The model under review builds one solid part; all positions refer to its coordinate system, in mm. A direction names the side the tool comes from. Round coordinates to 2 decimals unless told otherwise and drop trailing zeros. Order: outer loops, then holes, each group sorted by start corner. A loop starts at its lowest first (then second) coordinate and runs counter-clockwise, first axis right, second up. Notation, with made-up numbers: M 37.5,32.25 L 71.5,32.25 A24 ccw 71.5,53.25 Z; hole C 85,73 d9. An arc over 180 degrees is marked long. Answer as a JSON object with one key per item and string values. Group by question number.
1. Add section A-A on z = 5. State the section outline as (x, y) points, and give its area (3 significant figures).
2. Mouldability with a two-part tool opening along Z and no side actions: class faces 1 (the face through (-16.297, 39.418, 4.934)), 2 (the face through (-28.295, 36.978, 5.07)), 3 (the face through (-30.8, -25.9, 1.5)), 4 (the face through (-31.2, -24.2, 3.5)) as released by +Z, released by -Z, zero draft, split by the parting line, or undercut.
3. Machinability: for faces 5 (the face through (-30.8, -25.9, 8.5)), 6 (the face through (-29.799, 1, 5)), 7 (the face through (-31, -16.596, 5)), which of the approach directions +Z, -Z, +X, -X, +Y, -Y give a long, thin tool a straight path to every point of the face, cutting with its end or side? Answer none if there is none.
4. To check wall thickness, follow probe 1 along X at (y, z) = (15, 4.25); probe 2 along Y at (x, z) = (-30, 2); probe 3 along Y at (x, z) = (-11.25, 1.5). State the ranges of each line that lie inside material, in increasing order. Write a range as [from, to].
5. Clearance check with flat-ended pins moving along their axes: P1, Ø0.6, axis at x = -30.5, y = -21, coming from the +Z side; P2, Ø1, axis at y = -9, z = 2, coming from the +X side; P3, Ø1, axis at x = -31, z = 4.5, coming from the -Y side. State where each tip first meets the part, or that it passes through.
6. Add section B-B on y = 9.5. State the section outline as (x, z) points.
7. Add section C-C on x = -9. State the section outline as (y, z) points, and give its area (3 significant figures).
```python
from build123d import *

# Parameters (mm, degrees)
Y_KSEKLIK_EKSTR_ZYON1_DEPTH = 10
IZIM2_W                     = 1.5
IZIM2_H                     = 11.454648232
IZIM2_W_2                   = 3
IZIM2_H_2                   = 15
KES_EKSTR_ZYON1_DEPTH       = 10
IZIM3_R                     = 0.5
KES_EKSTR_ZYON2_DEPTH       = 22
IZIM4_R                     = 1.5
KES_EKSTR_ZYON3_DEPTH       = 44
RADYUS1_R                   = 5
RADYUS2_R                   = 2


with BuildPart() as part:
    # Çizim1 → Yükseklik-Ekstrüzyon1 (new body)
    with BuildSketch(Plane.XY):
        Polygon((-4.798797212, 38.403805497), (-29.798797212, 38.403805497), (-29.798797212, -31.596194503), (-31.798797212, -31.596194503), (-31.798797212, 40.403805497), (-4.798797212, 40.403805497), align=None)
    extrude(amount=Y_KSEKLIK_EKSTR_ZYON1_DEPTH)

    # Çizim2 → Kes-Ekstrüzyon1 (cut)
    with BuildSketch(Plane(origin=(-29.798797212, 0, 0), x_dir=(0, 0, -1), z_dir=(1, 0, 0))):
        with Locations((-9.25, -25.868870387)):
            Rectangle(IZIM2_W, IZIM2_H)
        with Locations((-0.75, -25.868870387)):
            Rectangle(IZIM2_W, IZIM2_H)
        with Locations((-5, -24.096194503)):
            Rectangle(IZIM2_W_2, IZIM2_H_2)
    extrude(amount=-KES_EKSTR_ZYON1_DEPTH, mode=Mode.SUBTRACT)

    # Çizim3 → Kes-Ekstrüzyon2 (cut, symmetric)
    with BuildSketch(Plane.XY.offset(8.5)):
        with Locations((-30.798797212, -29.596194503)):
            Circle(IZIM3_R)
        with Locations((-30.798797212, -26.596194503)):
            Circle(IZIM3_R)
        with Locations((-30.798797212, -23.596194503)):
            Circle(IZIM3_R)
        with Locations((-30.798797212, -20.596194503)):
            Circle(IZIM3_R)
        with Locations((-30.798797212, -17.596194503)):
            Circle(IZIM3_R)
    extrude(amount=KES_EKSTR_ZYON2_DEPTH, both=True, mode=Mode.SUBTRACT)

    # Çizim4 → Kes-Ekstrüzyon3 (cut)
    with BuildSketch(Plane(origin=(0, 40.403805497, 0), x_dir=(1, 0, 0), z_dir=(0, 1, 0))):
        with Locations((-14.798797212, -5)):
            Circle(IZIM4_R)
    extrude(amount=-KES_EKSTR_ZYON3_DEPTH, mode=Mode.SUBTRACT)

    # Radyus1
    radyus1_edges = [part.edges().sort_by_distance(p)[0] for p in [
        (-29.798797212, 38.403805497, 5),
    ]]
    fillet(radyus1_edges, radius=RADYUS1_R)

    # Radyus2
    radyus2_edges = [part.edges().sort_by_distance(p)[0] for p in [
        (-31.798797212, 40.403805497, 5),
    ]]
    fillet(radyus2_edges, radius=RADYUS2_R)


solid = part.part
```
Recorded:
{
 "1": {"outline": "M -31.8,-16.6 L -29.8,-16.6 L -29.8,33.4 A5 cw -24.8,38.4 L -16.3,38.4 L -16.3,40.4 L -29.8,40.4 A2 ccw -31.8,38.4 Z; M -13.3,38.4 L -4.8,38.4 L -4.8,40.4 L -13.3,40.4 Z", "area": "163 mm²"},
 "2": {"face 1": "undercut", "face 2": "zero draft", "face 3": "released by -Z", "face 4": "undercut"},
 "3": {"face 5": "+Z, +X, -X, -Y", "face 6": "+Z, -Z, +X, -Y", "face 7": "+X, -X, -Y"},
 "4": {"probe 1": "x = [-31.8, -29.8]", "probe 2": "y = [-31.6, 40.39]", "probe 3": "y = [38.4, 40.4]"},
 "5": {"P1": "stops at z = 8.5", "P2": "stops at x = -29.8", "P3": "stops at y = -16.6"},
 "6": {"outline": "M -31.8,0 L -29.8,0 L -29.8,10 L -31.8,10 Z"},
 "7": {"outline": "M 38.4,0 L 40.4,0 L 40.4,10 L 38.4,10 Z", "area": "20.0 mm²"}
}
